Build history of the part. All positions in model axes, mm. A direction names the side the tool comes from. Round coordinates to 2 decimals unless told otherwise and drop trailing zeros. Write each loop counter-clockwise with the first axis right and the second up, starting at its lowest first coordinate (ties: lowest second). Pieces come first, ordered by that corner, then holes. Notation, with made-up numbers: (-11.75, 8) - (39.25, 8) arc R25 cw to (39.25, 32) - close; hole circle Ø2 at (79, -5.75). An arc over 180 degrees is marked (long way). One line per question, with ' | ' between items.
Autodesk Inventor part; units mm, degrees
ref_plane "YZ Plane" through (0, 0, 0) normal (1, 0, 0) x (0, 1, 0)
ref_plane "XZ Plane" through (0, 0, 0) normal (0, 1, 0) x (-1, 0, 0)
ref_plane "XY Plane" through (0, 0, 0) normal (0, 0, 1) x (1, 0, 0)
sketch "Sketch1" plane through (0, 0, 0) normal (1, 0, 0) x (0, 1, 0)
  circle A0 centre (0, 0) radius 30.15
  dimension "d0" = 60.3
extrude "Extrude1" add sketch "Sketch1" along normal blind 128
sketch "Sketch2" plane through (0, 0, 0) normal (0, 0, 1) x (1, 0, 0)
  line L0 (0, 30.15) -> (0, -30.15)
  line L1 (128, 30.15) -> (128, -30.15)
  line L2 (0, 0) -> (128, 0) construction
  circle A0 centre (64, 0) radius 30.15
  dimension "d3" = 60.3
extrude "Extrude2" add sketch "Sketch2" along normal blind 64
sketch "Sketch3" plane through (0, 0, 0) normal (-1, 0, 0) x (0, 0, 1)
  circle A0 centre (0, 0) radius 30.15
  circle A1 centre (0, 0) radius 25.65
  dimension "d6" = 51.3
extrude "Extrude3" cut sketch "Sketch3" against normal through all contours A1
sketch "Sketch4" plane through (64, 0, 64) normal (0, 0, 1) x (1, 0, 0)
  circle A0 centre (0, 0) radius 30.15
  circle A1 centre (0, 0) radius 25.65
  dimension "d9" = 51.3
extrude "Extrude4" cut sketch "Sketch4" against normal up to next contours A1
equation "\"d0\" = d"
equation "\"d1\" = 2 * a"
equation "\"d3\" = d"
equation "\"d4\" = a"
equation "\"d6\" = d - 2 * s1"
equation "\"d7\" = a"
equation "\"d9\" = d - 2 * s1"
equation "\"d10\" = a"
equation "\"d\" = 60.3"
equation "\"s1\" = 4.5"
equation "\"a\" = 64"
equation "\"Size_Designation\" = 1.2345"
properties part number "DIN 2615-1 Tee 60.3 x 4 S" material "Steel"
Q1. Which spindle directions (+Z, -Z, +X, -X, +Y, -Y) get a long thin tool onto all of the face, cutting with end or side? Do faces 5 (the cylindrical face through (63.104, -3.925, -29.893)), 6 (the flat face through (73, 25, 64)). Say none if no direction does.
Found:
face 5: none | face 6: +Z, +X, -X, +Y, -Y
Q2. Saw through at D-D, the plane z = 38.5. List the corners of the cut face in (x, y), then the cut area to 3 significant figures.
Found:
outline: circle Ø60.3 at (64, 0); hole circle Ø51.3 at (64, 0) | area: 789 mm^2
Q3. Pull direction Y, two halves, no side cores. Call faces 1 (the cylindrical face through (77.79, 21.63, 39.56)), 2 (the cylindrical face through (33.88, -1.33, 38.66)), 3 (the flat face through (128, 9, 25)), 4 (the cylindrical face through (63.104, 1.128, -25.625)): +Y half, -Y half, draft (parallel to the pull), parting line (faces both ways), or undercut.
Found:
face 1: undercut | face 2: parting line | face 3: draft | face 4: undercut
Q4. Saw through at C-C, the plane x = 64. List the corners of the cut face in (y, z), then the cut area to 3 significant figures.
Found:
outline: (-30.15, 0) arc R30.15 ccw to (30.15, 0) - (30.15, 64) - (25.65, 64) - (25.65, 0) arc R25.65 cw to (-25.65, 0) - (-25.65, 64) - (-30.15, 64) - close | area: 970 mm^2
Q5. Saw through at A-A, the plane y = 0. List the corners of the cut face in (x, z), then the cut area to 3 significant figures.
Found:
outline: (0, -30.15) - (128, -30.15) - (128, -25.65) - (0, -25.65) - close; (0, 25.65) - (38.35, 25.65) - (38.35, 64) - (33.85, 64) - (33.85, 30.15) - (0, 30.15) - close; (89.65, 25.65) - (128, 25.65) - (128, 30.15) - (94.15, 30.15) - (94.15, 64) - (89.65, 64) - close | area: 1,230 mm^2
Q6. Drop flat-ended pins along their axis: pin 1 (2 mm diameter, centred on x = 91, z = -3, fed in from -Y); pin 2 (4 mm diameter, centred on x = 66.5, y = 7.5, fed in from -Z); pin 3 (8 mm diameter, centred on x = 112, z = -13, fed in from -Y). Give the stop position or say it passes through.
Found:
pin 1: y = -30.08 | pin 2: z = -29.64 | pin 3: y = -28.78
Q7. Saw through at B-B, the plane z = -15. List the corners of the cut face in (x, y), then the cut area to 3 significant figures.
Found:
outline: (0, -26.15) - (128, -26.15) - (128, -20.81) - (0, -20.81) - close; (0, 20.81) - (128, 20.81) - (128, 26.15) - (0, 26.15) - close | area: 1,370 mm^2
Q8. Drill centre lines: L1, parallel to Y at x = 64, z = 35; L2, parallel to X at y = 0, z = 48; L3, parallel to Y at x = 56, z = 49.5. Where is each one in solid material? Low to high. Write a range as from..to.
Found:
L1: -30.15..-25.65, 25.65..30.15 | L2: 33.85..38.35, 89.65..94.15 | L3: -29.07..-24.37, 24.37..29.07
